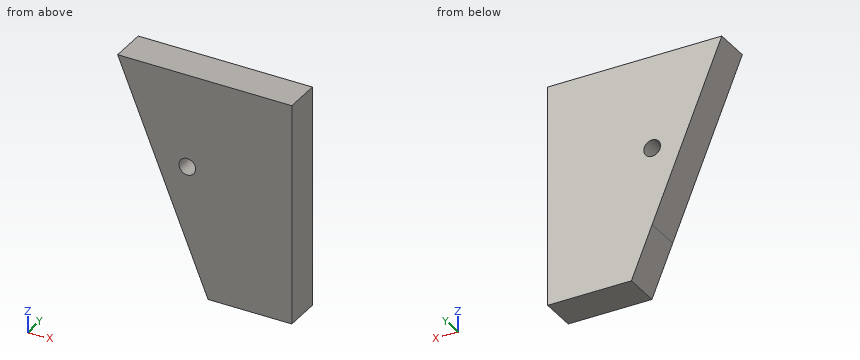
```python
from build123d import *

# Parameters (mm, degrees)
F1_DEPTH = 3.429


with BuildPart() as f1:
    # F0 (on Front) → F1 (new body, symmetric)
    with BuildSketch(Plane.XZ):
        Polygon((20.6095185396, -24.8038658976), (20.6095185396, 17.2331341024), (-12.4104814604, 17.2331341024), (0.7975185396, -15.1509251569), (4.7345185396, -24.8038658976), align=None)
        with BuildLine():
            ThreePointArc((2.3850185396, -0.4198658976), (1.9200505547, -1.5423979128), (0.7975185396, -2.0073658976))
            ThreePointArc((0.7975185396, -2.0073658976), (-0.3250134755, 0.7026661175), (2.3850185396, -0.4198658976))
        make_face(mode=Mode.SUBTRACT)
    extrude(amount=F1_DEPTH, both=True)


solid = f1.part
```
Can you work these out from the model? Positions are in its coordinate system, mm. Coordinates: 2 decimals unless noted, no trailing zeros. Write each loop counter-clockwise with the first axis right and the second up, starting at its lowest first coordinate (ties: lowest second). Pieces come first, ordered by that corner, then holes. Notation, with made-up numbers: M 28.5,71.5 L 39.5,71.5 A19 ccw 39.5,95.5 Z; hole C -34.5,-23 d2. An arc over 180 degrees is marked long. Answer as CSV lines item,"result".
Item 1: Please list where these lines run through material, in increasing order: line 1 along Z through (x, y) = (-0.5, -1.25); line 2 along X through (y, z) = (0.75, -11.5); line 3 along X through (y, z) = (-2.25, -18).
Geometry results:
line 1,"z = -11.97 to -1.33, 0.49 to 17.23"
line 2,"x = -0.69 to 20.61"
line 3,"x = 1.96 to 20.61"
Item 2: Imagine slicing it at B-B on z = -8. List the corners of the cut face in (x, y) for me, plus the area to 3 significant figures.
Geometry results:
outline,"M -2.12,-3.43 L 20.61,-3.43 L 20.61,3.43 L -2.12,3.43 Z"
area,"156 mm2"
Item 3: Imagine slicing it at A-A on y = -2.25. List the corners of the cut face in (x, z) for me (1 decimal).
Geometry results:
outline,"M -12.4,17.2 L 4.7,-24.8 L 20.6,-24.8 L 20.6,17.2 Z; hole C 0.8,-0.4 d3.2"
Item 4: Imagine slicing it at C-C on x = -3.5. List the corners of the cut face in (y, z) for me.
Geometry results:
outline,"M -3.43,-4.61 L 3.43,-4.61 L 3.43,17.23 L -3.43,17.23 Z"
Item 5: I'm going to push a flat-ended pin straight in: P1, Ø2, axis at y = 0.5, z = -16, coming from the -X side. Where does the tip first touch, or does it pass through?
Geometry results:
P1,"stops at x = 0.74"
